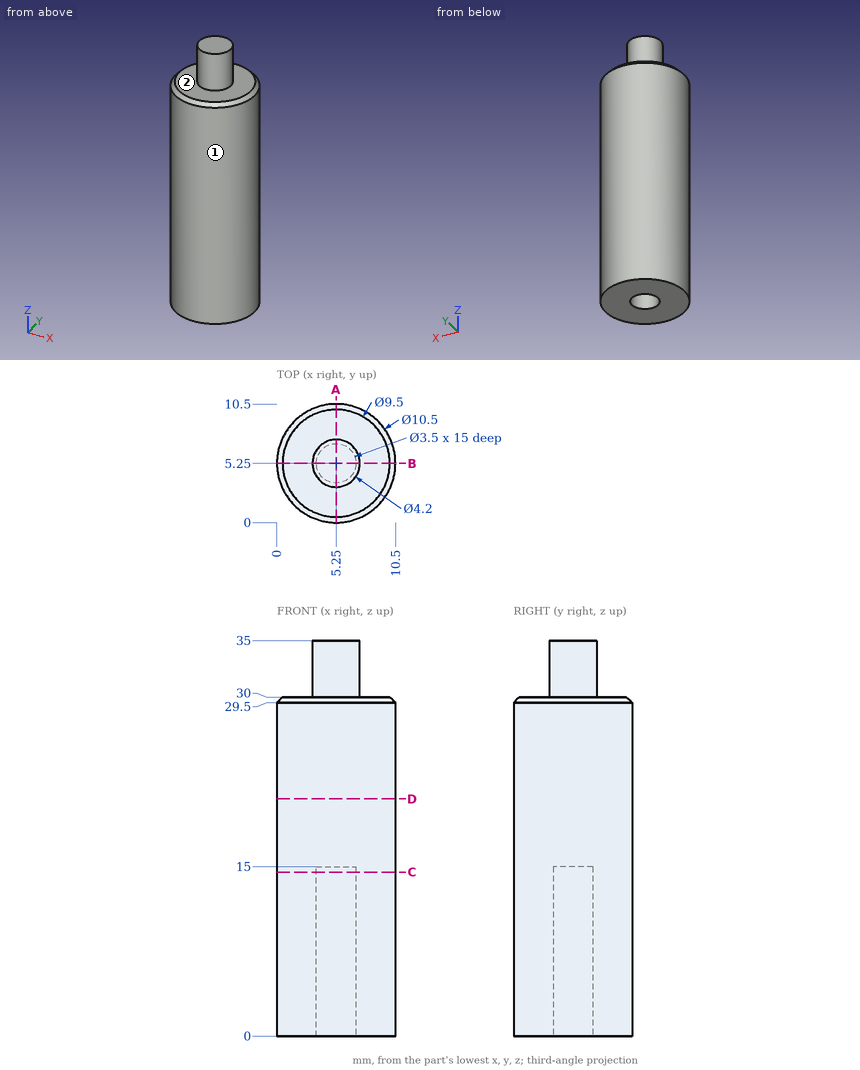
Can you work these out from the drawing? Everything is in mm from the part's minimum corner. A direction names the side the tool comes from. Coordinates: 2 decimals unless noted, no trailing zeros. Loops run counter-clockwise (first coordinate to the right, second up) from the corner with the lowest first, then second, coordinate; pieces in that order, holes last. Notation, with made-up numbers: (-27, -4) - (22, -4) arc R15 ccw to (22, 7) - close; hole circle Ø10 at (52, 43.5). An arc over 180 degrees is marked (long way). Use a Markdown table: item, result.
Item 1: I want a section at C-C on z = 14.5. Please give me the cut outline in (x, y), and give its area (3 significant figures).
Numbers:
| item | result |
|---|---|
| outline | circle Ø10.5 at (5.25, 5.25); hole circle Ø3.5 at (5.25, 5.25) |
| area | 77.0 mm2 |
Item 2: I want a section at A-A on x = 5.25. Please give me the cut outline in (y, z).
Numbers:
| item | result |
|---|---|
| outline | (0, 0) - (3.5, 0) - (3.5, 15) - (7, 15) - (7, 0) - (10.5, 0) - (10.5, 29.5) - (10, 30) - (7.35, 30) - (7.35, 35) - (3.15, 35) - (3.15, 30) - (0.5, 30) - (0, 29.5) - close |
Item 3: For the marked faces 1 and 2, which set-ups out of +Z, -Z, +X, -X, +Y, -Y let a thin tool reach every point of the face, with its end or its side?
Numbers:
| item | result |
|---|---|
| face 1 | +Z, -Z |
| face 2 | +Z |
Item 4: If I drill on probe 1 along Y at (x, z) = (5.25, 4.5); probe 2 along Z at (x, y) = (8.5, 8.25); probe 3 along Y at (x, z) = (7.5, 25.5), over which ranges is the centre line in solid material (lowest first)? Write a range as from..to.
Numbers:
| item | result |
|---|---|
| probe 1 | y = 0..3.5, 7..10.5 |
| probe 2 | z = 0..30 |
| probe 3 | y = 0.51..9.99 |
Item 5: Will these pins go through, and if not, where does the flat tip stop? pin 1 (3 mm diameter, centred on x = 7, z = 20.5, fed in from +Y); pin 2 (2 mm diameter, centred on x = 9.5, y = 2, fed in from +Z); pin 3 (6 mm diameter, centred on y = 1.5, z = 15, fed in from -X).
Numbers:
| item | result |
|---|---|
| pin 1 | stops at y = 10.49 |
| pin 2 | stops at z = 30 |
| pin 3 | stops at x = 0.05 |
Item 6: I want a section at D-D on z = 21. Please give me the cut outline in (x, y).
Numbers:
| item | result |
|---|---|
| outline | circle Ø10.5 at (5.25, 5.25) |
